```python
from build123d import *

# Parameters (mm, degrees)
F0_W     = 57
F0_H     = 57
F1_DEPTH = 2134


with BuildPart() as f1:
    # F0 (on Right) → F1 (new body)
    with BuildSketch(Plane.YZ):
        with BuildLine():
            Line((16.53541, 46.006598), (-37.46459, 46.006598))
            ThreePointArc((-37.46459, 46.006598), (-41.000124, 44.542132), (-42.46459, 41.006598))
            Line((-42.46459, 41.006598), (-42.46459, -12.993402))
            ThreePointArc((-42.46459, -12.993402), (-41.000124, -16.528936), (-37.46459, -17.993402))
            Line((-37.46459, -17.993402), (16.53541, -17.993402))
            ThreePointArc((16.53541, -17.993402), (20.070944, -16.528936), (21.53541, -12.993402))
            Line((21.53541, -12.993402), (21.53541, 41.006598))
            ThreePointArc((21.53541, 41.006598), (20.070944, 44.542132), (16.53541, 46.006598))
        make_face()
        with Locations((-10.46459, 14.006598)):
            Rectangle(F0_W, F0_H, mode=Mode.SUBTRACT)
    extrude(amount=F1_DEPTH)


solid = f1.part
```
Part model, mm, in its own coordinate system. A direction names the side the tool comes from. Round coordinates to 2 decimals unless told otherwise and drop trailing zeros. Order: outer loops, then holes, each group sorted by start corner. A loop starts at its lowest first (then second) coordinate and runs counter-clockwise, first axis right, second up. Notation, with made-up numbers: M -9,7.25 L 14,7.25 A5 cw 14,13.25 Z; hole C 6,21 d1. An arc over 180 degrees is marked long. Answer in a Markdown table with one row per item. Add a question column.
Q1. Mould opens along Z. For faces 1 (the face through (1052, -38.965, 14)), 2 (the face through (2134, -13, 43)), 3 (the face through (1052, -10, 46.007)) say: +Z half, -Z half, draft (parallel to the pull), parting line (faces both ways), or undercut.
Q2. Cut at C-C on y = -17.5. Give the cut face in (x, z), and give its area (3 significant figures).
Q3. Wall check: L1, parallel to Y at x = 999, z = 38; L2, parallel to Z at x = 1183, y = -5; L3, parallel to Z at x = 1716.5, y = 17.5. Give the ranges that are in metal, low to high. Write a range as from..to.
Q4. Cut at A-A on z = 9.5. Give the cut face in (x, y), and give its area (3 significant figures).
Q5. 3-axis set-ups, long thin cutter, end or side, ignore diameter. For faces 4 (the face through (1052, 21.535, 14)), 5 (the face through (1052, -11, -14.493)): which of +Z, -Z, +X, -X, +Y, -Y reach the whole face in a straight line?
Q6. Cut at B-B on x = 175. Give the cut face in (y, z), and give its area (3 significant figures).
Established:
| question | item | result |
|---|---|---|
| 1 | face 1 | undercut |
| 1 | face 2 | draft |
| 1 | face 3 | +Z half |
| 2 | outline | M 0,-17.99 L 2134,-17.99 L 2134,-14.49 L 0,-14.49 Z; M 0,42.51 L 2134,42.51 L 2134,46.01 L 0,46.01 Z |
| 2 | area | 14,900 mm2 |
| 3 | L1 | y = -42.46..-38.96, 18.04..21.54 |
| 3 | L2 | z = -17.99..-14.49, 42.51..46.01 |
| 3 | L3 | z = -17.9..-14.49, 42.51..45.91 |
| 4 | outline | M 0,-42.46 L 2134,-42.46 L 2134,-38.96 L 0,-38.96 Z; M 0,18.04 L 2134,18.04 L 2134,21.54 L 0,21.54 Z |
| 4 | area | 14,900 mm2 |
| 5 | face 4 | +Z, -Z, +X, -X, +Y |
| 5 | face 5 | +X, -X |
| 6 | outline | M -42.46,-12.99 A5 ccw -37.46,-17.99 L 16.54,-17.99 A5 ccw 21.54,-12.99 L 21.54,41.01 A5 ccw 16.54,46.01 L -37.46,46.01 A5 ccw -42.46,41.01 Z; hole M -38.96,-14.49 L 18.04,-14.49 L 18.04,42.51 L -38.96,42.51 Z |
| 6 | area | 826 mm2 |
